Source: CAD feature listing. Evaluate the final solid. Frame: model axes, mm. A direction names the side the tool comes from. Give positions to 0.01 mm unless a question says otherwise; leave off trailing zeros. Loops run counter-clockwise (first coordinate to the right, second up) from the corner with the lowest first, then second, coordinate; pieces in that order, holes last. Notation, with made-up numbers: M 70.5,0 L 107.5,0 A8 ccw 107.5,13 Z; hole C 10.25,-16.5 d2. An arc over 180 degrees is marked long. Write item = value, one per line.
from build123d import *

# Parameters (mm, degrees)
SKETCH1_W           = 79.1
SKETCH1_H           = 17.5
SKETCH2_R           = 6
BOSS_EXTRUDE1_DEPTH = 10
FILLET2_R           = 0.5
SKETCH3_R           = 3
CUT_EXTRUDE3_DEPTH  = 3


with BuildPart() as part:
    # Sketch1 → Revolve1 (revolve)
    with BuildSketch(Plane.XY):
        with Locations((-13.391352503, -1.567164179)):
            Rectangle(SKETCH1_W, SKETCH1_H)
    revolve(axis=Axis((-52.941352503, 7.182835821, 0), (1, 0, 0)))

    # Sketch2 → Boss-Extrude1 (add)
    with BuildSketch(Plane.ZY.offset(52.941352503)):
        with Locations((0, 14.182835821)):
            Circle(SKETCH2_R)
    extrude(amount=BOSS_EXTRUDE1_DEPTH)

    # Fillet2
    fillet2_edges = [part.edges().sort_by_distance(p)[0] for p in [
        (-62.941352503, 14.182835821, -6),
    ]]
    fillet(fillet2_edges, radius=FILLET2_R)

    # Sketch3 → Cut-Extrude3 (cut)
    with BuildSketch(Plane.ZY.offset(62.941352503)):
        with Locations((0, 14.182835821)):
            Circle(SKETCH3_R)
    extrude(amount=-CUT_EXTRUDE3_DEPTH, mode=Mode.SUBTRACT)


solid = part.part
1. Cut plane D-D, the plane z = -7. Return the cut outline in (x, y), then the cut area to 3 significant figures.
Derived:
outline = M -52.94,-8.86 L 26.16,-8.86 L 26.16,23.22 L -52.94,23.22 Z
area = 2,540 mm²
2. First-contact query: pin 1 Ø3.5 at (y, z) = (14.18, 0) entering from -X; pin 2 Ø2 at (y, z) = (-4, 13) entering from -X; pin 3 Ø12 at (x, y) = (5.5, 16.5) entering from -Z. Flat tips, straight axial feed; report the tip coordinate or a pass-through.
Derived:
pin_1 = -59.94
pin_2 = -52.94
pin_3 = -17.18
3. Cut plane A-A, the plane z = 0. Return the cut outline in (x, y).
Derived:
outline = M -62.94,8.68 A0.5 ccw -62.44,8.18 L -52.94,8.18 L -52.94,-10.32 L 26.16,-10.32 L 26.16,24.68 L -52.94,24.68 L -52.94,20.18 L -62.44,20.18 A0.5 ccw -62.94,19.68 L -62.94,17.18 L -59.94,17.18 L -59.94,11.18 L -62.94,11.18 Z
4. Pull-direction query (Z, two-part tool) for faces 1 (the flat face through (-59.941, 14, 0)), 2 (the cylindrical face through (-61.462, 17.157, -0.391)), 3 (the cylindrical face through (-12.84, 21.07, 10.65)), 4 (the flat face through (-62.941, 11.8, 2.4)); classes: +Z half, -Z half, draft (parallel to the pull), parting line (faces both ways), or undercut.
Derived:
face_1 = undercut
face_2 = undercut
face_3 = parting line
face_4 = draft
5. Cut plane C-C, the plane y = -6. Return the cut outline in (x, z), then the cut area to 3 significant figures.
Derived:
outline = M -52.94,-11.51 L 26.16,-11.51 L 26.16,11.51 L -52.94,11.51 Z
area = 1,820 mm²
6. Material intervals for probe 1 along Y at (x, z) = (-62, 0); probe 2 along X at (y, z) = (0.5, 10.5); probe 3 along Z at (x, y) = (-16.5, 4), sorted ascending. Write a range as from..to.
Derived:
probe_1 = 8.18..11.18, 17.18..20.18
probe_2 = -52.94..26.16
probe_3 = -17.21..17.21
7. Cut plane B-B, the plane x = -6.5. Return the cut outline in (y, z), then the cut area to 3 significant figures.
Derived:
outline = C 7.18,0 d35
area = 962 mm²
8. Reachability of faces 5 (the flat face through (26.159, 7, 0)), 6 (the cylindrical face through (-57.62, 20.13, -0.78)) from +Z, -Z, +X, -X, +Y, -Y: full face, straight path, thin tool, end or side. Return the list, or none.
Derived:
face_5 = +Z, -Z, +X, +Y, -Y
face_6 = -X
